```python
from build123d import *

# Parameters (mm, degrees)
SKETCH1_W           = 25
SKETCH1_H           = 35
BOSS_EXTRUDE1_DEPTH = 5
SKETCH2_W           = 9
SKETCH2_H           = 11
CUT_EXTRUDE1_DEPTH  = 6
SKETCH3_R           = 1.75
CUT_EXTRUDE2_DEPTH  = 6
SKETCH4_W           = 13
SKETCH4_H           = 20
SKETCH4_W_2         = 10
SKETCH4_H_2         = 16
BOSS_EXTRUDE2_DEPTH = 16


with BuildPart() as part:
    # Sketch1 → Boss-Extrude1 (new body)
    with BuildSketch(Plane.XY):
        with Locations((12.5, 17.5)):
            Rectangle(SKETCH1_W, SKETCH1_H)
    extrude(amount=BOSS_EXTRUDE1_DEPTH)

    # Sketch2 → Cut-Extrude1 (cut, through all)
    with BuildSketch(Plane.XY.offset(5)):
        with Locations((12.5, 17.5)):
            Rectangle(SKETCH2_W, SKETCH2_H)
    extrude(amount=-CUT_EXTRUDE1_DEPTH, mode=Mode.SUBTRACT)

    # Sketch3 → Cut-Extrude2 (cut, through all)
    with BuildSketch(Plane.XY.offset(5)):
        with Locations((3, 30.5)):
            Circle(SKETCH3_R)
        with Locations((3, 4.5)):
            Circle(SKETCH3_R)
        with Locations((22, 4.5)):
            Circle(SKETCH3_R)
        with Locations((22, 30.5)):
            Circle(SKETCH3_R)
    extrude(amount=-CUT_EXTRUDE2_DEPTH, mode=Mode.SUBTRACT)

    # Sketch4 → Boss-Extrude2 (add)
    with BuildSketch(Plane(origin=(0, 0, 0), x_dir=(-1, 0, 0), z_dir=(0, 0, -1))):
        with Locations((-12.5, 17.5)):
            Rectangle(SKETCH4_W, SKETCH4_H)
        with Locations((-12.5, 17.5)):
            Rectangle(SKETCH4_W_2, SKETCH4_H_2, mode=Mode.SUBTRACT)
    extrude(amount=BOSS_EXTRUDE2_DEPTH)


solid = part.part
```
CAD build for the part. Positions are in the model's coordinates, mm. A direction names the side the tool comes from. Round coordinates to 2 decimals unless told otherwise and drop trailing zeros. Loops run counter-clockwise (first coordinate to the right, second up) from the corner with the lowest first, then second, coordinate; pieces in that order, holes last. Notation, with made-up numbers: M 45.5,-9 L 90.5,-9 A20 cw 90.5,22 Z; hole C 65,-4.75 d7. An arc over 180 degrees is marked long. Use a Markdown table: item, result. Add a question column.
(1) Cut at A-A (x = 3). Give the cut face in (y, z).
(2) Drill centre lines: line 1 (Y direction, x = 22, z = 3.25); line 2 (Y direction, x = 10.25, z = -10.75); line 3 (X direction, y = 15, z = -6.5). Where is each one in solid material? Low to high.
(3) Cut at B-B (y = 4.5). Give the cut face in (x, z).
(4) Flat gauge pins, fed straight in: pin 1 (4 mm diameter, centred on x = 22, y = 30.5, fed in from -Z); pin 2 (5 mm diameter, centred on y = 14.5, z = -8, fed in from -X); pin 3 (5 mm diameter, centred on x = 10.5, z = -5.5, fed in from +Y); pin 4 (3 mm diameter, centred on x = 22, y = 4.5, fed in from -Z). Where does each tip first touch, or does it go through?
(5) Pull direction X, two halves, no side cores. Call faces 4 (the face through (6, 17, -8)), 5 (the face through (12, 0, 2)), 6 (the face through (20.25, 4.58, 2.54)), 7 (the face through (25, 17, 2)): +X half, -X half, draft (parallel to the pull), parting line (faces both ways), or undercut.
(6) Cut at C-C (z = -11.25). Give the cut face in (x, y), and give its area (3 significant figures).
(7) Cut at D-D (x = 12.5). Give the cut face in (y, z), and give its area (3 significant figures).
(8) Which spindle directions (+Z, -Z, +X, -X, +Y, -Y) get a long thin tool onto all of the face, cutting with end or side? Do faces 1 (the face through (12, 23, 3)), 2 (the face through (13, 27.5, -8)), 3 (the face through (7.7, 18.1, 0)). Say none if no direction does.
Geometry says:
| question | item | result |
|---|---|---|
| 1 | outline | M 0,0 L 2.75,0 L 2.75,5 L 0,5 Z; M 6.25,0 L 28.75,0 L 28.75,5 L 6.25,5 Z; M 32.25,0 L 35,0 L 35,5 L 32.25,5 Z |
| 2 | line 1 | y = 0 to 2.75, 6.25 to 28.75, 32.25 to 35 |
| 2 | line 2 | y = 7.5 to 9.5, 25.5 to 27.5 |
| 2 | line 3 | x = 6 to 7.5, 17.5 to 19 |
| 3 | outline | M 0,0 L 1.25,0 L 1.25,5 L 0,5 Z; M 4.75,0 L 20.25,0 L 20.25,5 L 4.75,5 Z; M 23.75,0 L 25,0 L 25,5 L 23.75,5 Z |
| 4 | pin 1 | stops at z = 0 |
| 4 | pin 2 | stops at x = 6 |
| 4 | pin 3 | stops at y = 27.5 |
| 4 | pin 4 | passes through |
| 5 | face 4 | -X half |
| 5 | face 5 | draft |
| 5 | face 6 | undercut |
| 5 | face 7 | +X half |
| 6 | outline | M 6,7.5 L 19,7.5 L 19,27.5 L 6,27.5 Z; hole M 7.5,9.5 L 17.5,9.5 L 17.5,25.5 L 7.5,25.5 Z |
| 6 | area | 100 mm² |
| 7 | outline | M 0,0 L 7.5,0 L 7.5,-16 L 9.5,-16 L 9.5,0 L 12,0 L 12,5 L 0,5 Z; M 23,0 L 25.5,0 L 25.5,-16 L 27.5,-16 L 27.5,0 L 35,0 L 35,5 L 23,5 Z |
| 7 | area | 184 mm² |
| 8 | face 1 | +Z, -Z |
| 8 | face 2 | -Z, +X, -X, +Y |
| 8 | face 3 | -Z |
